from build123d import *

# Parameters (mm, degrees)
SKETCH1_R           = 47.85
BOSS_EXTRUDE1_DEPTH = 222.25
SKETCH2_R           = 47.75
BOSS_EXTRUDE2_DEPTH = 183.95
FILLET1_R           = 47.85
SHELL1_T            = -5


with BuildPart() as part:
    # Sketch1 → Boss-Extrude1 (new body)
    with BuildSketch(Plane.XY):
        Circle(SKETCH1_R)
    extrude(amount=BOSS_EXTRUDE1_DEPTH)

    # Sketch2 → Boss-Extrude2 (add)
    with BuildSketch(Plane(origin=(0, 183.95, 0), x_dir=(1, 0, 0), z_dir=(0, 1, 0))):
        with Locations(Location((0, -60, 0), (0, 0, 270))):
            Circle(SKETCH2_R)
    extrude(amount=-BOSS_EXTRUDE2_DEPTH)

    # Sketch5 → Revolve3 (revolve)
    with BuildSketch(Plane(origin=(0, 0, 0), x_dir=(0, 0, -1), z_dir=(1, 0, 0)), mode=Mode.PRIVATE) as revolve3_sk:
        Polygon((-60, 183.95), (-12.25, 183.95), (-6.025, 189.95), (-6.025, 199.95), (-60, 199.95), align=None)
    revolve(revolve3_sk.sketch.rotate(Axis((0, 199.95, 60), (0, -1, 0)), 180), axis=Axis((0, 199.95, 60), (0, -1, 0)))

    # Fillet1
    fillet1_edges = [part.edges().sort_by_distance(p)[0] for p in [
        (-47.85, 0, 222.25),
    ]]
    fillet(fillet1_edges, radius=FILLET1_R)

    # Shell1
    shell1_openings = [part.faces().sort_by_distance(p)[0] for p in [
        (0, 199.95, 60),
        (0, 0, 0),
    ]]
    offset(amount=SHELL1_T, openings=shell1_openings, kind=Kind.INTERSECTION)


solid = part.part
Design review of the part built by this model. Coordinates are the model's own, in mm. A direction names the side the tool comes from. Coordinates: 2 decimals unless noted, no trailing zeros. Loops run counter-clockwise (first coordinate to the right, second up) from the corner with the lowest first, then second, coordinate; pieces in that order, holes last. Notation, with made-up numbers: (55.5, 51) -> (74.5, 51) arc R15 ccw to (74.5, 57) -> close; hole circle Ø1 at (-39, 68.5). An arc over 180 degrees is marked (long way). Use a Markdown table: item, result. Add a question column.
Item 1: We need section B-B, the plane z = 60. Write out the cut boundary in (x, y) (3 decimals).
Item 2: The part is to be moulded in two halves that separate along Z. For faces 1 (the flat face through (48, 199.95, 72)), 2 (the conical face through (16.52, 186.45, 99.85)), 3 (the cylindrical face through (-33.1, 196.068, 23.903)), 4 (the conical face through (-2.117, 184.325, 11.907)), say which applies: +Z half, -Z half, draft (parallel to the pull), parting line (faces both ways), or undercut.
Item 3: Wall thickness on L1, parallel to X at y = 197.5, z = 60 (3 decimals); L2, parallel to Y at x = 1.5, z = 174; L3, parallel to Y at x = -2, z = 184.5: over which ranges is each line inside the solid? List them lowest first. Write a range as from..to.
Item 4: We need section D-D, the plane y = 66.5. Write out the cut boundary in (x, z), and give its area (3 significant figures).
Item 5: We need section C-C, the plane y = 37. Write out the cut boundary in (x, z).
Item 6: We need section A-A, the plane x = 0. Write out the cut boundary in (y, z) (3 decimals).
Item 7: Clearance check with flat-ended pins moving along their axes: P1, Ø4, axis at y = 108.5, z = 54.5, coming from the +X side; P2, Ø12, axis at x = 39.5, z = 114, coming from the -Y side; P3, Ø12, axis at x = -17.5, z = 129.5, coming from the +Y side. State where each tip first meets the part, or that it passes through.
Item 8: Machinability: for faces 5 (the cylindrical face through (-9.29, -41.83, 85.98)), 6 (the cylindrical face through (14.343, 114.876, 105.545)), 7 (the cylindrical face through (1.88, 116.13, 17.29)), which of the approach directions +Z, -Z, +X, -X, +Y, -Y give a long, thin tool a straight path to every point of the face, cutting with its end or side? Answer none if there is none.
Numbers:
| question | item | result |
|---|---|---|
| 1 | outline | (-53.975, 189.95) -> (-47.75, 183.95) -> (-47.75, 3.092) arc R47.85 ccw (long way) to (47.75, 3.092) -> (47.75, 183.95) -> (53.975, 189.95) -> (53.975, 199.95) -> (48.975, 199.95) -> (48.975, 192.075) -> (42.75, 186.075) -> (42.75, 2.926) arc R42.85 cw (long way) to (-42.75, 2.926) -> (-42.75, 186.075) -> (-48.975, 192.075) -> (-48.975, 199.95) -> (-53.975, 199.95) -> close |
| 2 | face 1 | draft |
| 2 | face 2 | undercut |
| 2 | face 3 | undercut |
| 2 | face 4 | parting line |
| 3 | L1 | x = -53.975..-48.975, 48.975..53.975 |
| 3 | L2 | y = -47.83..-42.82, 42.82..47.83 |
| 3 | L3 | y = -46.73..-41.59, 41.59..46.73 |
| 4 | outline | circle Ø95.5 at (0, 60); hole circle Ø85.5 at (0, 60) |
| 4 | area | 1,420 mm^2 |
| 5 | outline | (-30.34, 0) -> (-21.61, 0) -> (-21.61, 23.12) arc R42.75 cw to (-21.61, 96.88) -> (-21.61, 174.4) arc R21.61 cw to (21.61, 174.4) -> (21.61, 96.88) arc R42.75 cw to (21.61, 23.12) -> (21.61, 0) -> (30.34, 0) -> (30.34, 23.13) arc R47.75 ccw to (30.34, 96.87) -> (30.34, 174.4) arc R30.34 ccw to (-30.34, 174.4) -> (-30.34, 96.87) arc R47.75 ccw to (-30.34, 23.13) -> close |
| 6 | outline | (-47.85, 0) -> (-42.85, 0) -> (-42.85, 174.4) arc R42.85 cw to (42.85, 174.4) -> (42.85, 102.75) -> (186.075, 102.75) -> (192.075, 108.975) -> (199.95, 108.975) -> (199.95, 113.975) -> (189.95, 113.975) -> (183.95, 107.75) -> (47.85, 107.75) -> (47.85, 174.4) arc R47.85 ccw to (-47.85, 174.4) -> close; (42.85, 0) -> (47.85, 0) -> (47.85, 12.25) -> (183.95, 12.25) -> (189.95, 6.025) -> (199.95, 6.025) -> (199.95, 11.025) -> (192.075, 11.025) -> (186.075, 17.25) -> (42.85, 17.25) -> close |
| 7 | P1 | stops at x = 47.62 |
| 7 | P2 | stops at y = -34.17 |
| 7 | P3 | stops at y = 46.45 |
| 8 | face 5 | -Z |
| 8 | face 6 | none |
| 8 | face 7 | +Y |
